```python
from build123d import *

# Parameters (mm, degrees)
F0_R     = 4
F1_DEPTH = 3
F5_DEPTH = 3
F8_DEPTH = 25
F9_DEPTH = 25


# Not quite as in the source:
# - ends of sketch curves that miss each other by under 0.0002 mm in the source are joined


with BuildPart() as f1:
    # F0 (on Front) → F1 (new body)
    with BuildSketch(Plane.XZ):
        with BuildLine():
            ThreePointArc((585.5387718609, -70.1653972109), (584.1001986375, -63.1555680907), (591.1100276795, -61.716994486))
            Line((591.1100276795, -61.716994486), (620.6688569888, -81.2094156242))
            Line((620.6688569888, -81.2094156242), (1035.0006136748, -147.2807863546))
            ThreePointArc((1035.0006136748, -147.2807863546), (1046.8897667562, -112.3036113444), (1076.917388022, -133.8232928895))
            Line((1076.917388022, -133.8232928895), (1516.7807656982, 301.1320483365))
            Line((1516.7807656982, 301.1320483365), (1482.3585617346, 388.849064))
            Line((1482.3585617346, 388.849064), (878.7694007197, 388.849064))
            Line((878.7694007197, 388.849064), (572.7458963991, -54.0303683051))
            ThreePointArc((572.7458963991, -54.0303683051), (569.563169725, -71.6485447179), (582.0179839674, -84.5096290961))
            Line((582.0179839674, -84.5096290961), (601.192342, -91.021836))
            ThreePointArc((601.192342, -91.021836), (606.4892645676, -88.6748164062), (605.0838007766, -83.0542683087))
            Line((605.0838007766, -83.0542683087), (585.5387718609, -70.1653972109))
        make_face()
        with Locations((1065.920517, -70.202665)):
            Circle(F0_R, mode=Mode.SUBTRACT)
        with Locations((926.6393642448, 354.4944504476)):
            Circle(F0_R, mode=Mode.SUBTRACT)
        with Locations((1472.9055166245, 338.570445776)):
            Circle(F0_R, mode=Mode.SUBTRACT)
    extrude(amount=F1_DEPTH)


with BuildPart() as f3_1:
    # F3: instance of F1
    add(f1.part.mirror(Plane(origin=(1180.5639812271, -1.5, 404.749064), x_dir=(1, 0, 0), z_dir=(0, 0, 1))))


with BuildPart() as f1_1:
    add(f1.part)

    add(f3_1.part)  # F5 merges F3_1
    # F4 (on face) → F5 (join, through all)
    with BuildSketch(Plane.XZ.offset(3)):
        with BuildLine():
            ThreePointArc((1473.8185102428, 388.849064), (1467.2383092365, 404.749064), (1473.8185102428, 420.649064))
            Line((1473.8185102428, 420.649064), (891.5892198284, 420.649064))
            ThreePointArc((891.5892198284, 420.649064), (901.7789530754, 404.749064), (891.5892198284, 388.849064))
            Line((891.5892198284, 388.849064), (1473.8185102428, 388.849064))
        make_face()
    extrude(amount=-F5_DEPTH)

    # F7 (on face) → F8 (cut)
    with BuildSketch(Plane.XZ.offset(3)):
        with BuildLine():
            Line((949.1413939246, -22.7795250632), (829.1413939246, -21.0615598373))
            ThreePointArc((829.1413939246, -21.0615598373), (811.3926761125, -38.3092558002), (828.6403720754, -56.0579736122))
            Line((828.6403720754, -56.0579736122), (948.6403720754, -57.7759388381))
            ThreePointArc((948.6403720754, -57.7759388381), (966.3890898875, -40.5282428752), (949.1413939246, -22.7795250632))
        make_face()
    extrude(amount=-F8_DEPTH, mode=Mode.SUBTRACT)

    # F6 (on face) → F9 (cut)
    with BuildSketch(Plane.XZ.offset(3)):
        with BuildLine():
            ThreePointArc((891.5892198284, 388.849064), (901.7789530754, 404.749064), (891.5892198284, 420.649064))
            Line((891.5892198284, 420.649064), (872.8003346685, 429.2875396296))
            Line((872.8003346685, 429.2875396296), (872.8003346685, 380.2105883704))
            Line((872.8003346685, 380.2105883704), (891.5892198284, 388.849064))
        make_face()
        with BuildLine():
            Line((1484.726747317, 382.814291443), (1484.726747317, 426.683836557))
            ThreePointArc((1484.726747317, 426.683836557), (1467.2383092365, 404.749064), (1484.726747317, 382.814291443))
        make_face()
    extrude(amount=-F9_DEPTH, mode=Mode.SUBTRACT)


solid = f1_1.part
```
Could you check a few things on this model? Use its own coordinates, in mm. A direction names the side the tool comes from. Round coordinates to 2 decimals unless told otherwise and drop trailing zeros. Loops run counter-clockwise (first coordinate to the right, second up) from the corner with the lowest first, then second, coordinate; pieces in that order, holes last. Notation, with made-up numbers: (33.5, -5.5) -> (65.5, -5.5) arc R22 cw to (65.5, 12.5) -> close; hole circle Ø10 at (86, 69.25). An arc over 180 degrees is marked (long way). Put each result on its own line as item: value.
Q1. Which directions (+Z, -Z, +X, -X, +Y, -Y) give clear straight access to the entire face, cutting with the end or side of a thin tool? Please do faces 1 (the cylindrical face through (1046.3, -1.5, 922)), 2 (the flat face through (1500.98, -1.48, 341.4)), 3 (the flat face through (724.873, -1.479, 166.13)).
Checks:
face 1: +Y, -Y
face 2: +X, +Y, -Y
face 3: -X, +Y, -Y
Q2. For pin 1 Ø7 at (x, z) = (1065.92, 879.7) entering from -Y; pin 2 Ø1 at (x, y) = (1175, -2) entering from -Z; pin 3 Ø10.5 at (x, z) = (1472.91, 338.57) entering from -Y, each with a flat end and sliding along its axis, tell me the tip position at first contact or that it passes through.
Checks:
pin 1: through
pin 2: z = -37.33
pin 3: y = -3
Q3. I want a section at D-D on x = 1050. Write out the boundary of the cut face in (y, z).
Checks:
outline: (-3, -111.54) -> (0, -111.54) -> (0, 921.04) -> (-3, 921.04) -> close
Q4. I want a section at A-A on x = 711. Write out the boundary of the cut face in (y, z).
Checks:
outline: (-3, -95.61) -> (0, -95.61) -> (0, 146.05) -> (-3, 146.05) -> close; (-3, 663.45) -> (0, 663.45) -> (0, 905.11) -> (-3, 905.11) -> close
Q5. Please list where these lines run through material, in increasing order: line 1 (Z direction, x = 856, y = -2.65); line 2 (Z direction, x = 927.5, y = -1.05); line 3 (X direction, y = -1, z = 873.5). Write a range as from..to.
Checks:
line 1: -118.74..-56.45, -21.45..355.9, 453.6..928.23
line 2: -130.14..-57.47, -22.47..350.59, 358.4..451.1, 458.91..939.64
line 3: 568.81..583.65, 594.57..1147.53
Q6. I want a section at B-B on y = -0.7. Give the number of separate pieces and of enclosed holes in the cut face, and give its area (3 significant figures).
Checks:
separate pieces: 1
enclosed holes: 7
area: 646,000 mm2
Q7. Thinking about a two-plate mould opening in X: for faces 4 (the flat face through (1293.77, -1.48, 728.89)), 5 (the flat face through (724.87, -1.48, 643.37)), 6 (the cylindrical face through (1046.3, -1.5, -112.5)), which applies, pulls with the +X half, pulls with the -X half, needs draft (parallel to the pull), parting line crosses it, or undercut?
Checks:
face 4: pulls with the +X half
face 5: pulls with the -X half
face 6: undercut
Q8. I want a section at C-C on z = 698. Write out the boundary of the cut face in (x, y), and give its area (3 significant figures).
Checks:
outline: (687.12, -3) -> (1325.01, -3) -> (1325.01, 0) -> (687.12, 0) -> close
area: 1,910 mm2
